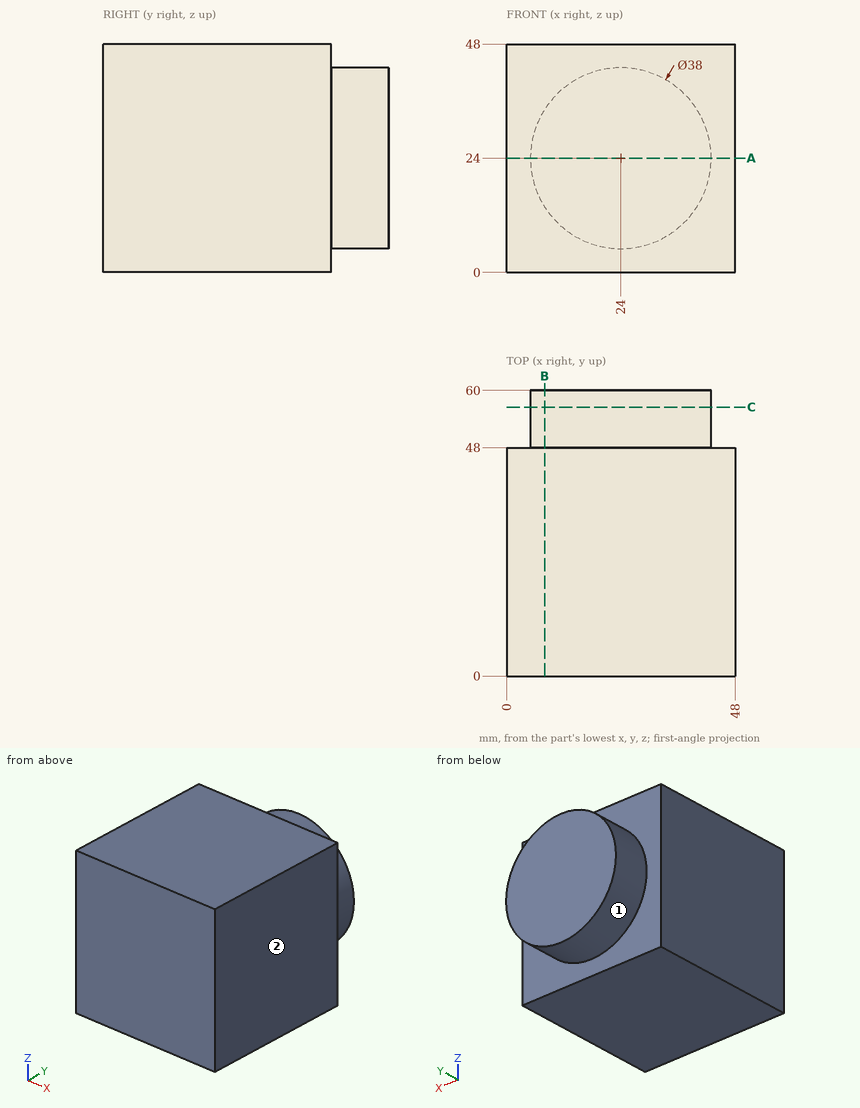
The drawing under review shows one solid part. Ordinate dimensions are in mm from its lowest x, y, z. A direction names the side the tool comes from. Coordinates: 2 decimals unless noted, no trailing zeros. Order: outer loops, then holes, each group sorted by start corner. A loop starts at its lowest first (then second) coordinate and runs counter-clockwise, first axis right, second up. Notation, with made-up numbers: M 55,11 L 70,11 A35 ccw 70,47 Z; hole C 45.25,46 d2. An arc over 180 degrees is marked long. One line per question, with ' | ' between items.
(1) Add section B-B, the plane x = 8. Write out the cut boundary in (y, z).
Geometry results:
outline: M 0,0 L 48,0 L 48,13.75 L 60,13.75 L 60,34.25 L 48,34.25 L 48,48 L 0,48 Z
(2) Machinability: for the marked faces 1 and 2, which of the approach directions +Z, -Z, +X, -X, +Y, -Y give a long, thin tool a straight path to every point of the face, cutting with its end or side? Answer none if there is none.
Geometry results:
face 1: +Y | face 2: +Z, -Z, +X, +Y, -Y
(3) For probe 1 along Y at (x, z) = (35, 6.5); probe 2 along Z at (x, y) = (8.5, 54); probe 3 along X at (y, z) = (56, 12), list the stretches that pass through material, from the lowest coordinate up. Write a range as from..to.
Geometry results:
probe 1: y = 0..48 | probe 2: z = 13.01..34.99 | probe 3: x = 9.27..38.73
(4) Add section C-C, the plane y = 56.5. Write out the cut boundary in (x, z).
Geometry results:
outline: C 24,24 d38
(5) Insertion check: pin 1 (4 mm diameter, centred on y = 25, z = 25.5, fed in from -X). The pin has a flat end and moves straight along its axis. Give the tip position at first contact, or say it passes through.
Geometry results:
pin 1: stops at x = 0
(6) Add section A-A, the plane z = 24. Write out the cut boundary in (x, y), then the cut area to 3 significant figures.
Geometry results:
outline: M 0,0 L 48,0 L 48,48 L 43,48 L 43,60 L 5,60 L 5,48 L 0,48 Z | area: 2,760 mm²
